```python
from build123d import *


with BuildPart() as f1:
    # F0 (on Front) → F1 (revolve)
    with BuildSketch(Plane.XZ):
        Polygon((-7, 2.95), (-7, 1.45), (0, 1.45), (0, 0.9), (6, 0.9), (6, 2.4), (1.952628, 2.4), (1, 2.4), (1, 2.95), align=None)
        Polygon((1.952628, 2.4), (1, 2.95), (1, 2.4), align=None)
    revolve(axis=Axis((-0.070939, 0, 0), (-1, 0, 0)))


solid = f1.part
```
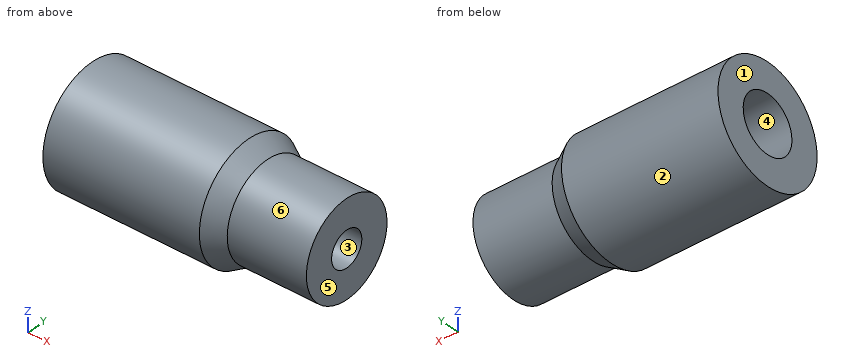
The listing builds one solid part. Answer for the finished solid, in the listing's coordinates (mm). Face numbers are marked on the shaded views. A direction names the side the tool comes from. Give positions to 0.01 mm unless a question says otherwise; leave off trailing zeros. Order: outer loops, then holes, each group sorted by start corner. A loop starts at its lowest first (then second) coordinate and runs counter-clockwise, first axis right, second up.
1) Determine the mould class of the marked faces 1, 2 and 3 for opening direction Y: pulls with the +Y half, pulls with the -Y half, needs draft (parallel to the pull), parting line crosses it, or undercut.
Reported:
face 1: needs draft
face 2: parting line crosses it
face 3: undercut
2) Find section C-C on x = -1.75. Write down the section's boundary in (y, z).
Reported:
outline: circle Ø5.9 at (0, 0); hole circle Ø2.9 at (0, 0)
3) For the marked faces 4, 5 and 6, determine the directions among +Z, -Z, +X, -X, +Y, -Y from which every point of the face is accessible in a straight line to the end or side of a thin tool.
Reported:
face 4: -X
face 5: +Z, -Z, +X, +Y, -Y
face 6: +X
4) Find section B-B on x = 3.5. Write down the section's boundary in (y, z), then the cut area to 3 significant figures.
Reported:
outline: circle Ø4.8 at (0, 0); hole circle Ø1.8 at (0, 0)
area: 15.6 mm2
5) Find section A-A on y = 0. Write down the section's boundary in (x, z), then the cut area to 3 significant figures.
Reported:
outline: (-7, -2.95) - (1, -2.95) - (1.95, -2.4) - (6, -2.4) - (6, -0.9) - (0, -0.9) - (0, -1.45) - (-7, -1.45) - close; (-7, 1.45) - (0, 1.45) - (0, 0.9) - (6, 0.9) - (6, 2.4) - (1.95, 2.4) - (1, 2.95) - (-7, 2.95) - close
area: 40.6 mm2
6) Consider line 1 along Y through (x, z) = (-5.5, 0); line 2 along Y through (x, z) = (4.5, 0); line 3 along X through (y, z) = (0.4, 1.05). Determine where each line is inside the solid, lowest interval first.
Reported:
line 1: y = -2.95 to -1.45, 1.45 to 2.95
line 2: y = -2.4 to -0.9, 0.9 to 2.4
line 3: x = 0 to 6
